from build123d import *

# Parameters (mm, degrees)
SKETCH1_R           = 7.5
BOSS_EXTRUDE1_DEPTH = 24
CHAMFER1_SIZE       = 0.4
FILLET2_R           = 3.175
SKETCH2_R           = 3.275
CUT_EXTRUDE1_DEPTH  = 50.405623415
CHAMFER2_SIZE       = 0.4
FILLET3_R           = 0.79375


with BuildPart() as part:
    # Sketch1 → Boss-Extrude1 (new body)
    with BuildSketch(Plane(origin=(0, 0, 0), x_dir=(1, 0, 0), z_dir=(0, 1, 0))):
        with BuildLine():
            Line((12.7, -6.35), (-12.7, -6.35))
            Line((-12.7, -6.35), (-12.7, 6.35))
            ThreePointArc((-12.7, 6.35), (-22.225, 15.875), (-12.7, 25.4))
            Line((-12.7, 25.4), (12.7, 25.4))
            ThreePointArc((12.7, 25.4), (22.225, 15.875), (12.7, 6.35))
            Line((12.7, 6.35), (12.7, -6.35))
        make_face()
        with Locations(Location((-12.7, 15.875, 0), (0, 0, 270))):
            Circle(SKETCH1_R, mode=Mode.SUBTRACT)
        with Locations(Location((12.7, 15.875, 0), (0, 0, 90))):
            Circle(SKETCH1_R, mode=Mode.SUBTRACT)
    extrude(amount=BOSS_EXTRUDE1_DEPTH)

    # Chamfer1
    chamfer1_edges = [part.edges().sort_by_distance(p)[0] for p in [
        (-12.7, 0, -23.375),
        (-12.7, 24, -23.375),
        (12.7, 0, -8.375),
        (12.7, 24, -8.375),
    ]]
    chamfer(chamfer1_edges, length=CHAMFER1_SIZE)

    # Fillet2
    fillet2_edges = [part.edges().sort_by_distance(p)[0] for p in [
        (0, 24, 6.35),
    ]]
    fillet(fillet2_edges, radius=FILLET2_R)

    # Sketch2 → Cut-Extrude1 (cut, through all)
    with BuildSketch(Plane(origin=(12.7, 0, 0), x_dir=(0, 0, -1), z_dir=(1, 0, 0))):
        with Locations((0, 19.14375)):
            Circle(SKETCH2_R)
        with Locations((0, 4.85625)):
            Circle(SKETCH2_R)
    extrude(amount=-CUT_EXTRUDE1_DEPTH, mode=Mode.SUBTRACT)

    # Chamfer2
    chamfer2_edges = [part.edges().sort_by_distance(p)[0] for p in [
        (-12.7, 19.14375, 3.275),
        (12.7, 19.14375, 3.275),
        (-12.7, 4.85625, 3.275),
        (12.7, 4.85625, 3.275),
    ]]
    chamfer(chamfer2_edges, length=CHAMFER2_SIZE)

    # Fillet3
    fillet3_edges = [part.edges().sort_by_distance(p)[0] for p in [
        (22.225, 24, -15.875),
        (0, 24, -25.4),
        (-22.225, 24, -15.875),
        (0, 0, -25.4),
        (22.225, 0, -15.875),
        (-22.225, 0, -15.875),
    ]]
    fillet(fillet3_edges, radius=FILLET3_R)


solid = part.part
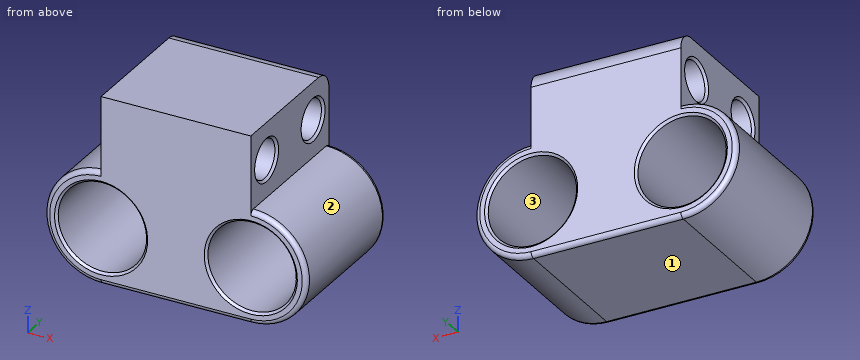
Work out the finished part from the listing and answer in its coordinate system (mm). Face numbers are marked on the shaded views. Round coordinates to 2 decimals unless told otherwise and drop trailing zeros. Write each loop counter-clockwise with the first axis right and the second up, starting at its lowest first coordinate (ties: lowest second). Pieces come first, ordered by that corner, then holes. Notation, with made-up numbers: (-28.75, 61.25) -> (-1.75, 61.25) arc R18 cw to (-1.75, 87.25) -> close; hole circle Ø8 at (33.25, -11.75). An arc over 180 degrees is marked (long way). Write each question's results on one line, items separated by ' | '.
Item 1: The mould has two halves that part along Z. Classify the marked faces 1, 2 and 3: +Z half, -Z half, draft (parallel to the pull), parting line (faces both ways), or undercut.
Result set:
face 1: -Z half | face 2: parting line | face 3: undercut
Item 2: Find the intervals of material crossed by line 1 along X through (y, z) = (5, -15.5); line 2 along Y through (x, z) = (2.25, 0); line 3 along X through (y, z) = (14.75, -13), in increasing order. Write a range as [from, to].
Result set:
line 1: [-22.22, -20.19], [-5.21, 5.21], [20.19, 22.22] | line 2: [0, 1.58], [8.13, 15.87], [22.42, 24] | line 3: [-21.78, -19.63], [-5.77, 5.77], [19.63, 21.78]
Item 3: A cutting plane is placed at A-A, the plane y = 14. Determine the outline of the cut face in (x, z) (3 decimals).
Result set:
outline: (-12.7, -25.4) -> (12.7, -25.4) arc R9.525 ccw to (12.7, -6.35) -> (12.7, 6.35) -> (-12.7, 6.35) -> (-12.7, -6.35) arc R9.525 ccw to start; hole circle Ø15 at (-12.7, -15.875); hole circle Ø15 at (12.7, -15.875)
Item 4: Flat-ended cylindrical pins translate along their axes: P1, Ø8.5, axis at y = 4.86, z = 0, coming from the -X side; P2, Ø1, axis at y = 14, z = -1.5, coming from the +X side; P3, Ø9, axis at x = 12.7, z = -15.875, coming from the -Y side; P4, Ø6, axis at y = 3.5, z = -5, coming from the -X side. Find the tip coordinate at first contact, or state that the pin passes through.
Result set:
P1: x = -12.7 | P2: x = 12.7 | P3: through | P4: x = -18.06
Item 5: A cutting plane is placed at C-C, the plane x = 0.5. Count the separate pieces of the cut face and the enclosed holes in it, plus the area to 3 significant figures.
Result set:
separate pieces: 1 | enclosed holes: 2 | area: 692 mm^2
Item 6: A cutting plane is placed at B-B, the plane z = 0. Determine the outline of the cut face in (x, y).
Result set:
outline: (-12.7, 0) -> (12.7, 0) -> (12.7, 1.18) -> (12.3, 1.58) -> (-12.3, 1.58) -> (-12.7, 1.18) -> close; (-12.7, 8.53) -> (-12.3, 8.13) -> (12.3, 8.13) -> (12.7, 8.53) -> (12.7, 15.47) -> (12.3, 15.87) -> (-12.3, 15.87) -> (-12.7, 15.47) -> close; (-12.7, 22.82) -> (-12.3, 22.42) -> (12.3, 22.42) -> (12.7, 22.82) -> (12.7, 24) -> (-12.7, 24) -> close
